Verification items for this drawing (mm, ordinates from the low corner). A direction names the side the tool comes from. Round coordinates to 2 decimals unless told otherwise and drop trailing zeros. Order: outer loops, then holes, each group sorted by start corner. A loop starts at its lowest first (then second) coordinate and runs counter-clockwise, first axis right, second up. Notation, with made-up numbers: (-35.75, 45) -> (16.25, 45) arc R29 ccw to (16.25, 73) -> close; hole circle Ø4 at (78.5, 75.5). An arc over 180 degrees is marked (long way). Use a Markdown table: item, result. Add a question column.
Item 1: Sectioned sample at A-A, the plane y = 12. Record the cut outline in (x, z) (1 decimal), and give its area (3 significant figures).
Item 2: Mould release check, pull along Z, two halves, no side actions. Record for the marked faces 1, 2 and 3: pulls with the +Z half, pulls with the -Z half, needs draft (parallel to the pull), parting line crosses it, or undercut.
Item 3: Gauge pin test, flat ends, axial feed: pin 1 Ø8 at (x, z) = (16.5, 13.5) entering from +Y; pin 2 Ø3 at (x, y) = (20.5, 6.5) entering from +Z; pin 3 Ø7.5 at (y, z) = (4, 14.5) entering from +X. Record the tip position at first contact, or that the pin passes through.
Item 4: Material ranges on probe 1 along X at (y, z) = (17, 5) (1 decimal); probe 2 along Y at (x, z) = (15.25, 18.75); probe 3 along X at (y, z) = (12.5, 13.5), recorded low to high. Write a range as [from, to].
Item 5: Set-up check for the marked faces 4, 5, 6, 7 and 8: record each of +Z, -Z, +X, -X, +Y, -Y from which the full face is reachable in a straight line by a thin tool's end or side.
Item 6: Sectioned sample at D-D, the plane z = 9. Record the cut outline in (x, y) (1 decimal).
Item 7: Sectioned sample at C-C, the plane x = 4.25. Record the cut outline in (y, z), and give its area (3 significant figures).
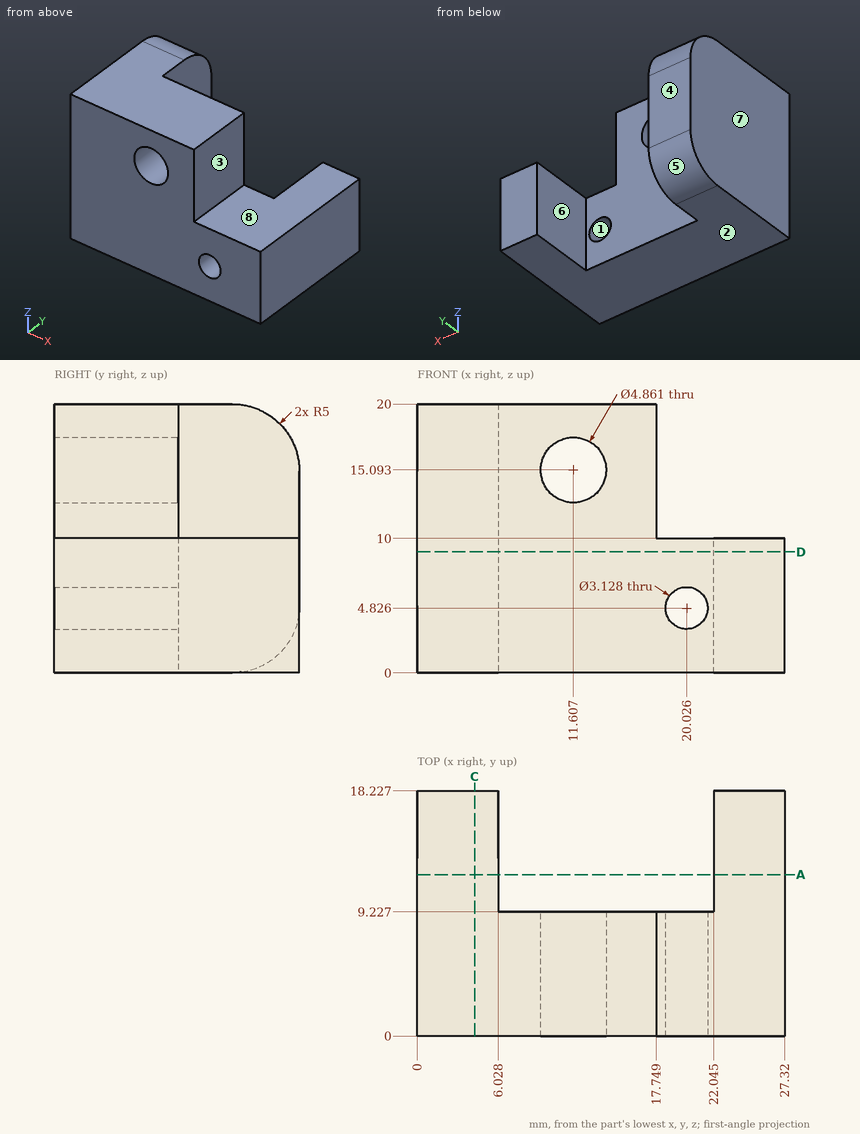
Found:
| question | item | result |
|---|---|---|
| 1 | outline | (0, 0) -> (6, 0) -> (6, 20) -> (0, 20) -> close; (22, 0) -> (27.3, 0) -> (27.3, 10) -> (22, 10) -> close |
| 1 | area | 173 mm2 |
| 2 | face 1 | undercut |
| 2 | face 2 | pulls with the -Z half |
| 2 | face 3 | needs draft |
| 3 | pin 1 | stops at y = 9.23 |
| 3 | pin 2 | stops at z = 10 |
| 3 | pin 3 | stops at x = 17.75 |
| 4 | probe 1 | x = [0, 6], [22, 27.3] |
| 4 | probe 2 | y = [0, 9.23] |
| 4 | probe 3 | x = [0, 6.03] |
| 5 | face 4 | +Z, -Z, +X, -X, +Y |
| 5 | face 5 | -Z, -X, +Y |
| 5 | face 6 | +Z, -Z, +Y |
| 5 | face 7 | +Z, -Z, -X, +Y, -Y |
| 5 | face 8 | +Z, +X, +Y, -Y |
| 6 | outline | (0, 0) -> (27.3, 0) -> (27.3, 18.2) -> (22, 18.2) -> (22, 9.2) -> (6, 9.2) -> (6, 18.2) -> (0, 18.2) -> close |
| 7 | outline | (0, 0) -> (13.23, 0) arc R5 ccw to (18.23, 5) -> (18.23, 15) arc R5 ccw to (13.23, 20) -> (0, 20) -> close |
| 7 | area | 354 mm2 |
